Work out the finished part from the listing and answer in its coordinate system (mm). Face numbers are marked on the shaded views. A direction names the side the tool comes from. Round coordinates to 2 decimals unless told otherwise and drop trailing zeros. Loops run counter-clockwise (first coordinate to the right, second up) from the corner with the lowest first, then second, coordinate; pieces in that order, holes last. Notation, with made-up numbers: (54.5, 72) -> (99.5, 72) arc R27 cw to (99.5, 94) -> close; hole circle Ø6 at (44.5, 29). An arc over 180 degrees is marked (long way). Use CSV: the item, a comma, the result in double quotes. Start each with the question number.
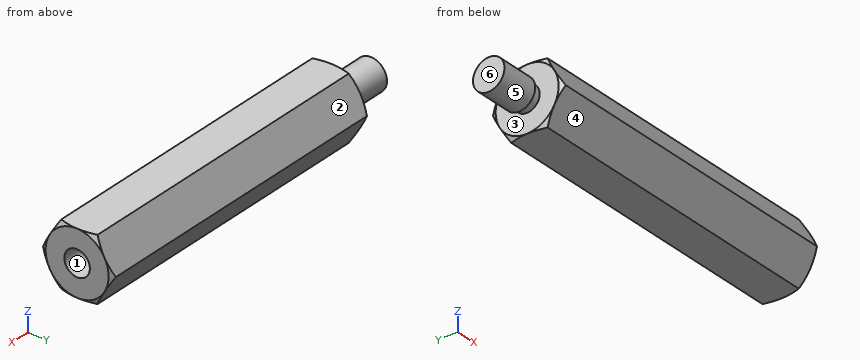
from build123d import *

# Parameters (mm, degrees)
BOSS_EXTRUDE1_DEPTH = 40
TAP4_D              = 3.242
TAP4_DEPTH          = 10.1
TAP4_TIP            = 0.973995063


with BuildPart() as part:
    # Sketch1 → Boss-Extrude1 (new body)
    with BuildSketch(Plane(origin=(0, 0, 0), x_dir=(0, 0, -1), z_dir=(1, 0, 0))):
        Polygon((0, 4.618802154), (-4, 2.309401077), (-4, -2.309401077), (0, -4.618802154), (4, -2.309401077), (4, 2.309401077), align=None)
    extrude(amount=BOSS_EXTRUDE1_DEPTH)

    # Sketch2 → Cut-Revolve1 (revolve, cut)
    with BuildSketch(Plane.XY):
        Polygon((0, 4.618802154), (0, 4), (0.35726559, 4.618802154), align=None)
        Polygon((39.64273441, 4.618802154), (40, 4.618802154), (40, 4), align=None)
    revolve(axis=Axis((0, 0, 0), (1, 0, 0)), mode=Mode.SUBTRACT)

    # Sketch11 → Revolve3 (revolve)
    with BuildSketch(Plane.XY):
        Polygon((0, 0), (0, 1.6), (-1.2, 1.6), (-1.2, 2), (-6, 2), (-6, 0), align=None)
    revolve(axis=Axis((0, 0, 0), (-1, 0, 0)))

    # Tap4
    with Locations(Plane(origin=(40, 0, 0), x_dir=(0, 0, -1), z_dir=(1, 0, 0))):
        with Locations((0, 0)):
            Hole(TAP4_D / 2, depth=TAP4_DEPTH)
            with Locations((0, 0, -(TAP4_DEPTH + TAP4_TIP / 2))):  # 118° drill point
                Cone(0, TAP4_D / 2, TAP4_TIP, mode=Mode.SUBTRACT)


solid = part.part
Q1. Section A-A, the plane x = 11 is taken. Write down the section's boundary in (y, z).
Q2. Which of the six approach directions +Z, -Z, +X, -X, +Y, -Y give full straight-line access (tool end or side, diameter ignored) to the marked faces 5 and 6?
Q3. Straight lines are drawn through the part: line 1 (Z direction, x = 37, y = 0); line 2 (Y direction, x = 32, z = 0); line 3 (X direction, y = 2.75, z = -0.25). For each, find the intervals that lie inside material, in ascending order. Write a range as from..to.
Q4. For a pull along Z with two mould halves and no side action, classify the marked faces 1, 2, 3 and 4 as pulls with the +Z half, pulls with the -Z half, needs draft (parallel to the pull), parting line crosses it, or undercut.
Report:
1,outline,"(-4.62, 0) -> (-2.31, -4) -> (2.31, -4) -> (4.62, 0) -> (2.31, 4) -> (-2.31, 4) -> close"
2,face 5,"-X"
2,face 6,"+Z, -Z, -X, +Y, -Y"
3,line 1,"z = -4..-1.62, 1.62..4"
3,line 2,"y = -4.62..-1.62, 1.62..4.62"
3,line 3,"x = 0..40"
4,face 1,"undercut"
4,face 2,"pulls with the +Z half"
4,face 3,"needs draft"
4,face 4,"pulls with the -Z half"
